Geometry check sheet. Reference: the model listing, model coordinates, mm. A direction names the side the tool comes from. Give positions to 0.01 mm unless a question says otherwise; leave off trailing zeros. Order: outer loops, then holes, each group sorted by start corner. A loop starts at its lowest first (then second) coordinate and runs counter-clockwise, first axis right, second up. Notation, with made-up numbers: M 25,-24.75 L 60,-24.75 A16 ccw 60,4.25 Z; hole C 14,32.5 d1. An arc over 180 degrees is marked long. Put each result on its own line as item: value. Start each with the question number.
Q1. Section check B-B on z = 1296.5. Record the cut outline in (x, y).
Q2. Mould release check, pull along X, two halves, no side actions. Record for faces 1 (the flat face through (489, 0, 983)), 2 (the flat face through (486, 150, 985)), 3 (the flat face through (35, 150, 985)): +X half, -X half, draft (parallel to the pull), parting line (faces both ways), or undercut.
Q3. Go/stop test with flat-tipped pins: pin 1 (3 mm diameter, centred on x = 405, z = 348, fed in from +Y); pin 2 (11 mm diameter, centred on x = 31, y = 5.5, fed in from -Z); pin 3 (3 mm diameter, centred on y = 154.5, z = 1238.5, fed in from -X). Record where each tip stops, or that it passes through.
Q4. Material ranges on L1, parallel to X at y = 80, z = 1155.5; L2, parallel to X at y = 218.5, z = 375.5; L3, parallel to Z at x = 256, y = 57.5, recorded low to high.
Q5. Section check D-D on z = 95. Record the cut outline in (x, y).
Q6. Access from +Z, -Z, +X, -X, +Y, -Y to the whole of each face (thin tool, end or side, straight path). Record for faces 4 (the flat face through (-4, 41, 461)), 5 (the flat face through (34, 226, 314)), 6 (the flat face through (8.5, 81, 124)), 7 (the flat face through (7.486, 45.49, 1527.286)), 8 (the flat face through (261, 95, 279)).
Q7. Section check A-A on x = 405. Record the cut outline in (y, z).
Q8. Section check C-C on y = 179.5. Record the cut outline in (x, z), then the cut area to 3 significant figures.
```python
from build123d import *

# Parameters (mm, degrees)
EXTRUDE_1_DEPTH        = 1992.775637732
EXTRUDE_1_2_DEPTH      = 1992.775637732
EXTRUDE_3_DEPTH        = 520
PATTERN_LINEAR_1_COUNT = 3
PATTERN_LINEAR_1_PITCH = 700
EXTRUDE_5_DEPTH        = 2
EXTRUDE_8_DEPTH        = 2
EXTRUDE_11_DEPTH       = 8.5
PATTERN_LINEAR_2_COUNT = 2
PATTERN_LINEAR_2_PITCH = 17
SKETCH_6_W             = 494.5
SKETCH_6_H             = 200
SKETCH_6_W_2           = 503
SKETCH_6_W_3           = 8.5
CUT_EXTRUDE_12_DEPTH   = 2066.709258908
SKETCH_20_R            = 24.25
CUT_EXTRUDE_13_DEPTH   = 2068.865322582
FILLET_1_R             = 40
SKETCH_21_W            = 8.5
SKETCH_21_H            = 225
EXTRUDE_14_DEPTH       = 175
SKETCH_22_R            = 22.25
CUT_EXTRUDE_15_DEPTH   = 2089.705817567
FILLET_2_R             = 175
FILLET_3_R             = 75
SKETCH_23_R            = 11
CUT_EXTRUDE_16_DEPTH   = 2089.198879915


with BuildPart() as part:
    # Sketch 2 → Extrude 1 (new body)
    with BuildSketch(Plane.XY):
        Polygon((0, 0), (0, 160), (63, 160), (63, 150), (6.5, 150), (6.5, 10), (63, 10), (63, 0), align=None)
    extrude(amount=EXTRUDE_1_DEPTH)



with BuildPart() as body_2:
    # Sketch 2 → Extrude 1 2 (new body)
    with BuildSketch(Plane.XY):
        Polygon((457, 160), (520, 160), (520, 0), (457, 0), (457, 10), (513.5, 10), (513.5, 150), (457, 150), align=None)
    extrude(amount=EXTRUDE_1_2_DEPTH)


with BuildPart() as part_1:
    add(part.part)

    add(body_2.part)  # Extrude 3 merges body 2
    # Sketch 5 → Extrude 3 (add)
    with BuildSketch(Plane.ZY):
        Polygon((200, 95), (360, 95), (360, 88.5), (283.25, 88.5), (283.25, 48.5), (276.75, 48.5), (276.75, 88.5), (200, 88.5), align=None)
    extrude_3 = extrude(amount=-EXTRUDE_3_DEPTH)

    # Pattern Linear 1: Extrude 3 ×3
    with Locations(*[(0, 0, i * PATTERN_LINEAR_1_PITCH) for i in range(1, PATTERN_LINEAR_1_COUNT)]):
        add(extrude_3)

    # Sketch 7 → Extrude 5 (add)
    with BuildSketch(Plane.ZY.offset(-513.5)):
        Polygon((0, 10), (500, 10), (570, 80), (500, 150), (0, 150), align=None)
        Polygon((1562.775637732, 150), (1492.775637732, 80), (1562.775637732, 10), (1992.775637732, 10), (1992.775637732, 150), align=None)
    extrude(amount=EXTRUDE_5_DEPTH)

    # Sketch 15 → Extrude 8 (add)
    with BuildSketch(Plane(origin=(6.5, 0, 0), x_dir=(0, 0, -1), z_dir=(1, 0, 0))):
        Polygon((-1992.775637732, 150), (-1562.775637732, 150), (-1492.775637732, 80), (-1562.775637732, 10), (-1992.775637732, 10), align=None)
        Polygon((-430, 150), (0, 150), (0, 10), (-430, 10), (-500, 80), align=None)
    extrude(amount=EXTRUDE_8_DEPTH)

    # Sketch 19 → Extrude 11 (add)
    with BuildSketch(Plane.ZY):
        Polygon((0, 160), (420, 160), (500, 80), (420, 0), (0, 0), align=None)
    extrude_11 = extrude(amount=EXTRUDE_11_DEPTH)

    # Pattern Linear 2: Extrude 11 ×2
    with Locations(*[(i * PATTERN_LINEAR_2_PITCH, 0, 0) for i in range(1, PATTERN_LINEAR_2_COUNT)]):
        add(extrude_11)

    # Sketch 6 → Cut-Extrude 12 (cut, through all)
    with BuildSketch(Plane(origin=(0, 160, 0), x_dir=(1, 0, 0), z_dir=(0, 1, 0))):
        with Locations((264.25, -100)):
            Rectangle(SKETCH_6_W, SKETCH_6_H)
        with Locations((260, -1892.775637732)):
            Rectangle(SKETCH_6_W_2, SKETCH_6_H)
        with Locations((4.25, -100)):
            Rectangle(SKETCH_6_W_3, SKETCH_6_H)
    extrude(amount=-CUT_EXTRUDE_12_DEPTH, mode=Mode.SUBTRACT)

    # Sketch 20 → Cut-Extrude 13 (cut, through all)
    with BuildSketch(Plane.ZY.offset(8.5)):
        with Locations((95, 80)):
            Circle(SKETCH_20_R)
        with Locations(Location((1897.775637732, 80, 0), (0, 0, 90))):
            Circle(SKETCH_20_R)
    extrude(amount=-CUT_EXTRUDE_13_DEPTH, mode=Mode.SUBTRACT)

    # Fillet 1
    fillet_1_edges = [part_1.edges().sort_by_distance(p)[0] for p in [
        (4.25, 0, 1992.775637732),
        (4.25, 160, 1992.775637732),
        (515.75, 0, 1992.775637732),
        (515.75, 160, 1992.775637732),
        (-4.25, 0, 0),
        (12.75, 0, 0),
        (-4.25, 160, 0),
        (12.75, 160, 0),
        (515.75, 0, 0),
        (515.75, 160, 0),
    ]]
    fillet(fillet_1_edges, radius=FILLET_1_R)

    # Sketch 21 → Extrude 14 (add)
    with BuildSketch(Plane(origin=(0, 160, 0), x_dir=(1, 0, 0), z_dir=(0, 1, 0))):
        with Locations((515.75, -312.5)):
            Rectangle(SKETCH_21_W, SKETCH_21_H)
        with Locations((12.75, -312.5)):
            Rectangle(SKETCH_21_W, SKETCH_21_H)
        with Locations((29.75, -312.5)):
            Rectangle(SKETCH_21_W, SKETCH_21_H)
    extrude(amount=EXTRUDE_14_DEPTH)

    # Sketch 22 → Cut-Extrude 15 (cut, through all)
    with BuildSketch(Plane.ZY.offset(8.5)):
        with Locations((344.615088301, 246.410058868)):
            Circle(SKETCH_22_R)
    extrude(amount=-CUT_EXTRUDE_15_DEPTH, mode=Mode.SUBTRACT)

    # Fillet 2
    fillet_2_edges = [part_1.edges().sort_by_distance(p)[0] for p in [
        (12.75, 335, 200),
        (515.75, 335, 200),
        (29.75, 335, 200),
    ]]
    fillet(fillet_2_edges, radius=FILLET_2_R - 0.0001)  # a hair under: the kernel refuses the full size

    # Fillet 3
    fillet_3_edges = [part_1.edges().sort_by_distance(p)[0] for p in [
        (12.75, 335, 425),
        (515.75, 335, 425),
        (29.75, 335, 425),
    ]]
    fillet(fillet_3_edges, radius=FILLET_3_R)

    # Sketch 23 → Cut-Extrude 16 (cut, through all)
    with BuildSketch(Plane(origin=(520, 0, 0), x_dir=(0, 0, -1), z_dir=(1, 0, 0))):
        with Locations((-1397.775637732, 80)):
            Circle(SKETCH_23_R)
        with Locations((-647.775637732, 80)):
            Circle(SKETCH_23_R)
    extrude(amount=-CUT_EXTRUDE_16_DEPTH, mode=Mode.SUBTRACT)


solid = part_1.part
```
Results found:
1. outline: M 0,0 L 63,0 L 63,10 L 6.5,10 L 6.5,150 L 63,150 L 63,160 L 0,160 Z; M 457,0 L 520,0 L 520,160 L 457,160 L 457,150 L 513.5,150 L 513.5,10 L 457,10 Z
2. face 1: draft
2. face 2: undercut
2. face 3: undercut
3. pin 1: stops at y = 95
3. pin 2: stops at z = 200
3. pin 3: stops at x = 0
4. L1: x = 0 to 6.5, 513.5 to 520
4. L2: x = 8.5 to 17, 25.5 to 34, 511.5 to 520
4. L3: z = 276.75 to 283.25, 976.75 to 983.25, 1676.75 to 1683.25
5. outline: M -8.5,0 L 0,0 L 0,55.75 L -8.5,55.75 Z; M -8.5,104.25 L 0,104.25 L 0,160 L -8.5,160 Z; M 8.5,0 L 17,0 L 17,55.75 L 8.5,55.75 Z; M 8.5,104.25 L 17,104.25 L 17,160 L 8.5,160 Z; M 511.5,0 L 520,0 L 520,55.75 L 511.5,55.75 Z; M 511.5,104.25 L 520,104.25 L 520,160 L 511.5,160 Z
6. face 4: +Z, -X, -Y
6. face 5: +Z, -Z, +Y
6. face 6: -Z, +Y, -Y
6. face 7: none
6. face 8: +Z, -Z
7. outline: M 48.5,276.75 L 88.5,276.75 L 88.5,200 L 95,200 L 95,360 L 88.5,360 L 88.5,283.25 L 48.5,283.25 Z; M 48.5,976.75 L 88.5,976.75 L 88.5,900 L 95,900 L 95,1060 L 88.5,1060 L 88.5,983.25 L 48.5,983.25 Z; M 48.5,1676.75 L 88.5,1676.75 L 88.5,1600 L 95,1600 L 95,1760 L 88.5,1760 L 88.5,1683.25 L 48.5,1683.25 Z
8. outline: M 8.5,201.09 L 17,201.09 L 17,425 L 8.5,425 Z; M 25.5,201.09 L 34,201.09 L 34,425 L 25.5,425 Z; M 511.5,201.09 L 520,201.09 L 520,425 L 511.5,425 Z
8. area: 5,710 mm^2
